Autodesk Inventor part; units mm, degrees
ref_plane "YZ Plane" through (0, 0, 0) normal (1, 0, 0) x (0, 1, 0)
ref_plane "XZ Plane" through (0, 0, 0) normal (0, 1, 0) x (-1, 0, 0)
ref_plane "XY Plane" through (0, 0, 0) normal (0, 0, 1) x (1, 0, 0)
sketch "Sketch1" plane through (0, 0, 0) normal (0, 0, 1) x (1, 0, 0)
  line L0 (-16.5, -15) -> (16.5, -15)
  line L1 (16.5, -15) -> (16.5, 15)
  line L2 (16.5, 15) -> (-16.5, 15)
  line L3 (-16.5, 15) -> (-16.5, -15)
  line L4 (-16.5, -15) -> (16.5, 15) construction
  line L5 (16.5, -15) -> (-16.5, 15) construction
  point P0 (0, 0)
  dimension "d0" = 33
  dimension "d1" = 30
extrude "Extrusion1" add sketch "Sketch1" along normal mid plane 100
sketch "Sketch2" plane through (0, 0, 50) normal (0, 0, 1) x (1, 0, 0)
  line L0 (10.7831, 13.1928) -> (16.3277, 0.3976)
  arc A0 (10.7831, 13.1928) -> (8.0304, 15) centre (8.0304, 12) ccw
  line L1 (8.0304, 15) -> (16.5, 15)
  line L2 (16.5, 15) -> (16.5, 0)
  line L3 (-10.7831, 13.1928) -> (-16.3277, 0.3976)
  arc A1 (-8.0304, 15) -> (-10.7831, 13.1928) centre (-8.0304, 12) ccw
  line L4 (-8.0304, 15) -> (-16.5, 15)
  line L5 (-16.5, 15) -> (-16.5, 0)
  line L6 (10.7831, -13.1928) -> (16.3277, -0.3976)
  arc A2 (8.0304, -15) -> (10.7831, -13.1928) centre (8.0304, -12) ccw
  line L7 (8.0304, -15) -> (16.5, -15)
  line L8 (16.5, -15) -> (16.5, 0)
  line L9 (-10.7831, -13.1928) -> (-16.3277, -0.3976)
  arc A3 (-10.7831, -13.1928) -> (-8.0304, -15) centre (-8.0304, -12) ccw
  line L10 (-8.0304, -15) -> (-16.5, -15)
  line L11 (-16.5, -15) -> (-16.5, 0)
  arc A4 (-16.3277, 0.3976) -> (-16.3277, -0.3976) centre (-15.4101, 0) ccw
  arc A5 (16.3277, -0.3976) -> (16.3277, 0.3976) centre (15.4101, 0) ccw
  point P0 (0, 0)
  point P1 (10, 15)
  point P2 (-10, 15)
  point P3 (10, -15)
  point P4 (-10, -15)
  dimension "d10" = 3
  dimension "d11" = 1
extrude "Extrusion2" cut sketch "Sketch2" against normal blind 100
properties part number "Powerbank"
Work out the finished part from the listing and answer in its coordinate system (mm). Coordinates: 2 decimals unless noted, no trailing zeros. Loops run counter-clockwise (first coordinate to the right, second up) from the corner with the lowest first, then second, coordinate; pieces in that order, holes last. Notation, with made-up numbers: (-33, 77) - (-20, 77) arc R23 cw to (-20, 113) - close; hole circle Ø4 at (68, -17.75). An arc over 180 degrees is marked (long way). Use a Markdown table: item, result.
Item 1: Find section C-C, the plane x = 13.5. Determine the outline of the cut face in (y, z), and give its area (3 significant figures).
Evaluation:
| item | result |
|---|---|
| outline | (-6.92, -50) - (6.92, -50) - (6.92, 50) - (-6.92, 50) - close |
| area | 1,380 mm2 |
Item 2: Find section B-B, the plane y = -1.75. Determine the outline of the cut face in (x, z).
Evaluation:
| item | result |
|---|---|
| outline | (-15.74, -50) - (15.74, -50) - (15.74, 50) - (-15.74, 50) - close |
Item 3: Consider probe 1 along Y at (x, z) = (14.5, 20); probe 2 along X at (y, z) = (10.5, 34.5); probe 3 along X at (y, z) = (6.75, 36.5). Determine where each line is inside the solid, lowest interval first. Write a range as from..to.
Evaluation:
| item | result |
|---|---|
| probe 1 | y = -4.62..4.62 |
| probe 2 | x = -11.95..11.95 |
| probe 3 | x = -13.57..13.57 |
Item 4: Given pin 1 Ø2 at (y, z) = (10.5, 34.5) entering from +X; pin 2 Ø4 at (y, z) = (-7.5, -18.5) entering from -X; pin 3 Ø1 at (y, z) = (5.5, 4) entering from -X, each flat-ended and moving along its own axis, determine where each tip first touches the part or whether it passes through.
Evaluation:
| item | result |
|---|---|
| pin 1 | stops at x = 12.38 |
| pin 2 | stops at x = -14.12 |
| pin 3 | stops at x = -14.33 |
Item 5: Find section A-A, the plane z = -7. Determine the outline of the cut face in (x, y), and give its area (3 significant figures).
Evaluation:
| item | result |
|---|---|
| outline | (-16.33, -0.4) - (-10.78, -13.19) arc R3 ccw to (-8.03, -15) - (8.03, -15) arc R3 ccw to (10.78, -13.19) - (16.33, -0.4) arc R1 ccw to (16.33, 0.4) - (10.78, 13.19) arc R3 ccw to (8.03, 15) - (-8.03, 15) arc R3 ccw to (-10.78, 13.19) - (-16.33, 0.4) arc R1 ccw to start |
| area | 792 mm2 |
